Part model, mm, in its own coordinate system. Coordinates: 2 decimals unless noted, no trailing zeros. Write each loop counter-clockwise with the first axis right and the second up, starting at its lowest first coordinate (ties: lowest second). Pieces come first, ordered by that corner, then holes. Notation, with made-up numbers: (-10, 89) - (41, 89) arc R27 cw to (41, 112) - close; hole circle Ø8 at (53.5, -9). An arc over 180 degrees is marked (long way). Use a Markdown table: item, result.
```python
from build123d import *

# Parameters (mm, degrees)
F0_W     = 101.6
F0_H     = 50.8
F1_DEPTH = 50.8
F3_DEPTH = 115.824
F5_DEPTH = 33.528
F6_DEPTH = 41.402


with BuildPart() as f1:
    # F0 (on Top) → F1 (new body)
    with BuildSketch(Plane.XY):
        with Locations((6.0652717948, 1.7450194966)):
            Rectangle(F0_W, F0_H)
    extrude(amount=F1_DEPTH)

    # F2 (on face) → F3 (cut)
    with BuildSketch(Plane(origin=(-44.7347282052, 0, 0), x_dir=(0, -1, 0), z_dir=(-1, 0, 0))):
        Polygon((-27.1450194966, 20.6477418542), (-1.7450194966, 50.8), (-27.1450194966, 50.8), align=None)
        Polygon((23.6549805034, 50.8), (-1.7450194966, 50.8), (23.6549805034, 20.6477418542), align=None)
    extrude(amount=-F3_DEPTH, mode=Mode.SUBTRACT)

    # F4 (on Front) → F5 (cut)
    with BuildSketch(Plane.XZ):
        Polygon((-21.6801278293, 51.361259073), (-44.908836484, 51.361259073), (-45.6831306219, 21.680129692), align=None)
        Polygon((57.2974830866, 51.361259073), (35.1011604071, 51.361259073), (57.2974830866, 21.680129692), align=None)
    extrude(amount=-F5_DEPTH, mode=Mode.SUBTRACT)

    # F6 (cut): faces of the model
    f6_faces = [f1.faces().sort_by_distance(p)[0] for p in [
        (50.2668517161, 0, 39.9050242048),
        (-37.7595636519, 0, 40.1032904014),
    ]]
    extrude(f6_faces, amount=-F6_DEPTH, mode=Mode.SUBTRACT)


solid = f1.part
```
Item 1: Band-saw the part on D-D, the plane x = 49. Give the cut face in (y, z).
From the geometry:
| item | result |
|---|---|
| outline | (-23.65, 0) - (27.15, 0) - (27.15, 20.65) - (16.93, 32.78) - (-13.44, 32.78) - (-23.65, 20.65) - close |
Item 2: Band-saw the part on B-B, the plane y = -15.5. Give the cut face in (x, z).
From the geometry:
| item | result |
|---|---|
| outline | (-44.73, 0) - (56.87, 0) - (56.87, 22.26) - (50.83, 30.33) - (-38.69, 30.33) - (-44.73, 22.85) - close |
Item 3: Drop flat-ended pins along their axis: P1, Ø10, axis at x = -14, z = 36.5, coming from the +Y side; P2, Ø12, axis at y = 8, z = 32.5, coming from the +X side. Give the stop position or say it passes through.
From the geometry:
| item | result |
|---|---|
| P1 | y = 18 |
| P2 | x = 53.69 |
Item 4: Band-saw the part on C-C, the plane z = 26.5. Give the cut face in (x, y).
From the geometry:
| item | result |
|---|---|
| outline | (-41.79, -18.73) - (53.69, -18.73) - (53.69, 22.22) - (-41.79, 22.22) - close |
Item 5: Band-saw the part on A-A, the plane x = 11. Give the cut face in (y, z).
From the geometry:
| item | result |
|---|---|
| outline | (-23.65, 0) - (27.15, 0) - (27.15, 20.65) - (1.75, 50.8) - (-23.65, 20.65) - close |
Item 6: Drill centre lines: probe 1 along Z at (x, y) = (-3.5, -3.5); probe 2 along Y at (x, z) = (35, 40.5); probe 3 along X at (y, z) = (2.5, 45). Where is each one in solid material? Low to high.
From the geometry:
| item | result |
|---|---|
| probe 1 | 0 to 44.57 |
| probe 2 | -6.93 to 10.42 |
| probe 3 | -26.82 to 39.86 |
